```python
from build123d import *

# Parameters (mm, degrees)
F0_R     = 1.08
F1_DEPTH = 15
F0_R_2   = 1.225
F2_DEPTH = 13.5
F0_R_3   = 1.75
F3_DEPTH = 4
F0_R_4   = 3.575
F4_DEPTH = 2.7


with BuildPart() as f1:
    # F0 (on Top) → F1 (new body)
    with BuildSketch(Plane.XY):
        Circle(F0_R)
    extrude(amount=F1_DEPTH)

    # F0 (on Top) → F2 (join)
    with BuildSketch(Plane.XY):
        Circle(F0_R_2)
        Circle(F0_R, mode=Mode.SUBTRACT)
    extrude(amount=F2_DEPTH)

    # F0 (on Top) → F3 (join)
    with BuildSketch(Plane.XY):
        Circle(F0_R_3)
        Circle(F0_R_2, mode=Mode.SUBTRACT)
    extrude(amount=F3_DEPTH)

    # F0 (on Top) → F4 (join)
    with BuildSketch(Plane.XY):
        Circle(F0_R_4)
        Circle(F0_R_3, mode=Mode.SUBTRACT)
    extrude(amount=F4_DEPTH)


solid = f1.part
```
Source: CAD feature listing. Evaluate the final solid. Frame: model axes, mm. A direction names the side the tool comes from. Coordinates: 2 decimals unless noted, no trailing zeros. Loops run counter-clockwise (first coordinate to the right, second up) from the corner with the lowest first, then second, coordinate; pieces in that order, holes last. Notation, with made-up numbers: M 55,-7 L 63,-7 A25 cw 63,24 Z; hole C -34.5,-8 d1. An arc over 180 degrees is marked long. Put each result on its own line as item: value. Start each with the question number.
1) Cut plane D-D on y = 3. Return the cut outline in (x, z).
2) Contact query for flat-ended pins moving along their axis: pin 1 Ø3 at (y, z) = (1, 10) entering from -X (3 decimals); pin 2 Ø1 at (x, z) = (0.5, 10.5) entering from +Y (3 decimals); pin 3 Ø1 at (x, y) = (-2.5, -1) entering from +Z. Output: stop coordinate, or through.
3) Cut plane A-A on y = 0. Return the cut outline in (x, z) (3 decimals).
4) Ray query, L1, parallel to Z at x = 1.25, y = 1.5; L2, parallel to Y at x = 2.5, z = 2.5; L3, parallel to X at y = 0.5, z = 5.5. Return the intervals inside material, ascending. Write a range as from..to.
5) Reachability of faces 1 (the face through (0, 0, 0)), 2 (the face through (-0.266, -1.196, 8.683)) from +Z, -Z, +X, -X, +Y, -Y: full face, straight path, thin tool, end or side. Return the list, or none.
6) Cut plane C-C on z = 13.25. Return the cut outline in (x, y) (3 decimals).
The answers:
1. outline: M -1.94,0 L 1.94,0 L 1.94,2.7 L -1.94,2.7 Z
2. pin 1: stops at x = -1.225
2. pin 2: stops at y = 1.225
2. pin 3: stops at z = 2.7
3. outline: M -3.575,0 L 3.575,0 L 3.575,2.7 L 1.75,2.7 L 1.75,4 L 1.225,4 L 1.225,13.5 L 1.08,13.5 L 1.08,15 L -1.08,15 L -1.08,13.5 L -1.225,13.5 L -1.225,4 L -1.75,4 L -1.75,2.7 L -3.575,2.7 Z
4. L1: z = 0..2.7
4. L2: y = -2.56..2.56
4. L3: x = -1.12..1.12
5. face 1: -Z, +X, -X, +Y, -Y
5. face 2: +Z
6. outline: C 0,0 d2.45
